Part model, mm, in its own coordinate system. A direction names the side the tool comes from. Coordinates: 2 decimals unless noted, no trailing zeros. Loops run counter-clockwise (first coordinate to the right, second up) from the corner with the lowest first, then second, coordinate; pieces in that order, holes last. Notation, with made-up numbers: (44.25, 13.25) - (98.25, 13.25) arc R22 cw to (98.25, 30.25) - close; hole circle Ø3 at (-36.75, 13). An arc over 180 degrees is marked (long way). Use a Markdown table: item, result. Add a question column.
1) Probe probe 1 along Z at (x, y) = (-1.5, 1.75); probe 2 along X at (y, z) = (4.5, 7); probe 3 along Z at (x, y) = (2.75, 4.25). List the from-to ranges inside material, lowest first. Write a range as [from, to].
2) Band-saw the part on C-C (x = 6). Give the cut face in (y, z).
3) Tool access for faces 1 (the face through (4.1, 1, -6.9)), 2 (the face through (4.45, 2.46, 7.85)): list every direction of +Z, -Z, +X, -X, +Y, -Y with a clear straight run to the whole face (end or side of a thin tool).
4) Band-saw the part on B-B (z = -3.25). Give the cut face in (x, y) (3 decimals).
5) Band-saw the part on A-A (y = 0.5). Give the cut face in (x, z) (3 decimals), plus the area to 3 significant figures.
6) Band-saw the part on D-D (y = 3). Give the cut face in (x, z) (3 decimals), plus the area to 3 significant figures.
7) Drop flat-ended pins along their axis: P1, Ø1, axis at x = -2, y = 3.5, coming from the -Z side; P2, Ø0.7, axis at x = -1, y = 0.5, coming from the +Z side; P3, Ø1.5, axis at x = 6, y = 4, coming from the -Z side. Give the stop position or say it passes through.
8) Pull direction X, two halves, no side cores. Call faces 3 (the face through (-4.45, 2.46, -7.85)), 4 (the face through (-1, -1.5, -1)), 5 (the face through (0, 0, -2.45)): +X half, -X half, draft (parallel to the pull), parting line (faces both ways), or undercut.
from build123d import *

# Parameters (mm, degrees)
BOSS_EXTRUDE1_DEPTH = 5
SHELL1_T            = -1
BOSS_EXTRUDE2_DEPTH = 2
SKETCH3_W           = 6.8
SKETCH3_H           = 4.9
BOSS_EXTRUDE3_DEPTH = 3.5
CUT_EXTRUDE1_DEPTH  = 3.5
CUT_EXTRUDE2_DEPTH  = 1


with BuildPart() as part:
    # Sketch1 → Boss-Extrude1 (new body)
    with BuildSketch(Plane(origin=(0, 0, 0), x_dir=(1, 0, 0), z_dir=(0, 1, 0))):
        Polygon((9.025, 5.210586179), (0, 10.421172359), (-9.025, 5.210586179), (-9.025, -5.210586179), (0, -10.421172359), (9.025, -5.210586179), align=None)
    extrude(amount=BOSS_EXTRUDE1_DEPTH)

    # Shell1
    shell1_openings = [part.faces().sort_by_distance(p)[0] for p in [
        (0, 0, 0),
    ]]
    offset(amount=SHELL1_T, openings=shell1_openings, kind=Kind.INTERSECTION)

    # Sketch2 → Boss-Extrude2 (add)
    with BuildSketch(Plane.XZ.offset(-4)):
        Polygon((8.025, -4.63323591), (8.025, 4.63323591), (0, 9.26647182), (-8.025, 4.63323591), (-8.025, -4.63323591), (0, -9.26647182), align=None)
    extrude(amount=BOSS_EXTRUDE2_DEPTH)

    # Sketch3 → Boss-Extrude3 (add)
    with BuildSketch(Plane.XZ.offset(-2)):
        Rectangle(SKETCH3_W, SKETCH3_H)
    extrude(amount=BOSS_EXTRUDE3_DEPTH)

    # Sketch4 → Cut-Extrude1 (cut)
    with BuildSketch(Plane.XZ.offset(1.5)):
        Polygon((2.1, -0.65), (2.1, 0.65), (0.75, 0.65), (0.75, 2.1), (-0.75, 2.1), (-0.75, 0.65), (-2.1, 0.65), (-2.1, -0.65), (-0.75, -0.65), (-0.75, -2.1), (0.75, -2.1), (0.75, -0.65), align=None)
    extrude(amount=-CUT_EXTRUDE1_DEPTH, mode=Mode.SUBTRACT)

    # Sketch5 → Cut-Extrude2 (cut)
    with BuildSketch(Plane(origin=(0, 5, 0), x_dir=(1, 0, 0), z_dir=(0, 1, 0))):
        Polygon((-4.981910893, -4.812655517), (7.063361543, 2.144475893), (8.375460902, -0.127158722), (-3.669811534, -7.084290132), align=None)
    extrude(amount=-CUT_EXTRUDE2_DEPTH, mode=Mode.SUBTRACT)


solid = part.part
Answer block:
| question | item | result |
|---|---|---|
| 1 | probe 1 | [-9.56, -8.4], [-2.45, -0.65], [0.65, 2.45], [8.4, 9.56] |
| 1 | probe 2 | [-5.93, -3.72], [-3.52, 5.93] |
| 1 | probe 3 | [-8.83, 0.35], [3.38, 8.83] |
| 2 | outline | (0, -6.96) - (5, -6.96) - (5, -1.53) - (4, -1.53) - (4, 1.5) - (5, 1.5) - (5, 6.96) - (0, 6.96) - (0, 5.8) - (2, 5.8) - (2, -5.8) - (0, -5.8) - close |
| 3 | face 1 | -Y |
| 3 | face 2 | +Z, +X, +Y, -Y |
| 4 | outline | (-9.025, 0) - (-8.025, 0) - (-8.025, 2) - (8.025, 2) - (8.025, 0) - (9.025, 0) - (9.025, 5) - (-9.025, 5) - close |
| 5 | outline | (-9.025, -5.211) - (0, -10.421) - (9.025, -5.211) - (9.025, 5.211) - (0, 10.421) - (-9.025, 5.211) - close; (-3.4, -2.45) - (3.4, -2.45) - (3.4, 2.45) - (-3.4, 2.45) - close; hole (-8.025, -4.633) - (0, -9.266) - (8.025, -4.633) - (8.025, 4.633) - (0, 9.266) - (-8.025, 4.633) - close; hole (-2.1, -0.65) - (-0.75, -0.65) - (-0.75, -2.1) - (0.75, -2.1) - (0.75, -0.65) - (2.1, -0.65) - (2.1, 0.65) - (0.75, 0.65) - (0.75, 2.1) - (-0.75, 2.1) - (-0.75, 0.65) - (-2.1, 0.65) - close |
| 5 | area | 82.6 mm2 |
| 6 | outline | (-9.025, -5.211) - (0, -10.421) - (9.025, -5.211) - (9.025, 5.211) - (0, 10.421) - (-9.025, 5.211) - close |
| 6 | area | 282 mm2 |
| 7 | P1 | z = -9.56 |
| 7 | P2 | z = 10.05 |
| 7 | P3 | z = -7.39 |
| 8 | face 3 | -X half |
| 8 | face 4 | draft |
| 8 | face 5 | undercut |
